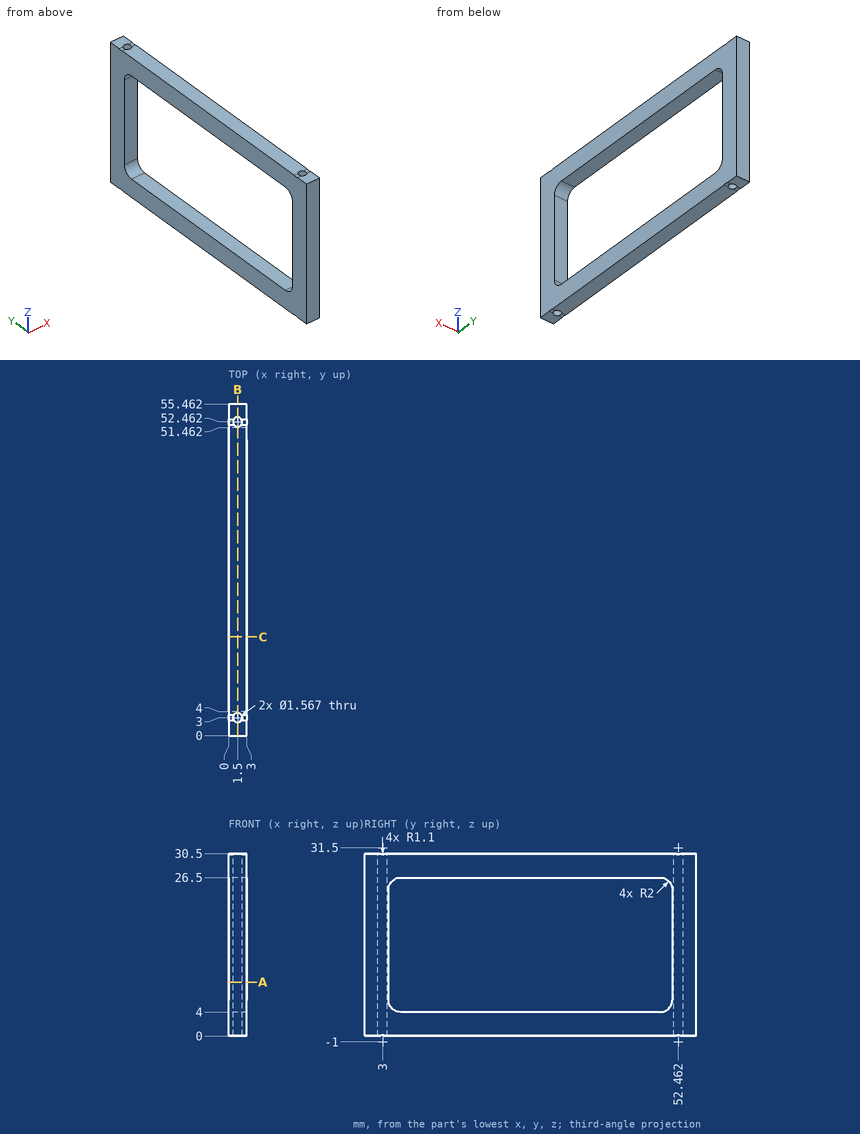
The figure shows three views and two pictorial views of one solid part (mm, origin at its lowest corner). Answer the questions. Round coordinates to 2 decimals unless told otherwise and drop trailing zeros. Loops run counter-clockwise (first coordinate to the right, second up) from the corner with the lowest first, then second, coordinate; pieces in that order, holes last. Notation, with made-up numbers: M 73,-10 L 116,-10 A35 ccw 116,26 Z; hole C 84,9.5 d3. An arc over 180 degrees is marked long. Write each question's results on one line, items separated by ' | '. Start each with the question number.
1) Find section A-A on z = 9. Write down the section's boundary in (x, y).
2) Straight lines are drawn through the part: probe 1 along X at (y, z) = (3, 14.5); probe 2 along Z at (x, y) = (2.2, 24); probe 3 along Y at (x, z) = (0.6, 20). For each, find the intervals that lie inside material, in ascending order.
3) Find section B-B on x = 1.5. Write down the section's boundary in (y, z).
4) This flat-tipped pin is pushed along its axis until it touches: pin 1 (0.9 mm diameter, centred on x = 1.5, y = 3, fed in from +Z). Where does it stop, or does it pass through?
5) Find section C-C on y = 16.5. Write down the section's boundary in (x, z).
Final values:
1) outline: M 0,0 L 3,0 L 3,4 L 0,4 Z; M 0,51.46 L 3,51.46 L 3,55.46 L 0,55.46 Z; hole C 1.5,3 d1.57; hole C 1.5,52.46 d1.57
2) probe 1: 0 to 0.72, 2.28 to 3 | probe 2: 0 to 4, 26.5 to 30.5 | probe 3: 0 to 4, 51.46 to 55.46
3) outline: M 0,0 L 2.22,0 L 2.22,30.5 L 0,30.5 Z; M 3.78,0 L 51.68,0 L 51.68,30.5 L 3.78,30.5 Z; M 53.25,0 L 55.46,0 L 55.46,30.5 L 53.25,30.5 Z; hole M 4,6 A2 ccw 6,4 L 49.46,4 A2 ccw 51.46,6 L 51.46,24.5 A2 ccw 49.46,26.5 L 6,26.5 A2 ccw 4,24.5 Z
4) pin 1: through
5) outline: M 0,0 L 3,0 L 3,4 L 0,4 Z; M 0,26.5 L 3,26.5 L 3,30.5 L 0,30.5 Z
